Geometry: final body of the model. Coordinates: model frame, mm. Face numbers are marked on the shaded views. A direction names the side the tool comes from. Coordinates: 2 decimals unless noted, no trailing zeros. Write each loop counter-clockwise with the first axis right and the second up, starting at its lowest first coordinate (ties: lowest second). Pieces come first, ordered by that corner, then holes. Notation, with made-up numbers: M -36.5,-38 L -10.5,-38 A25 ccw -10.5,-19 Z; hole C -18.75,31.5 d5. An arc over 180 degrees is marked long. Write item = value, one per line. Start each with the question number.
Item 1: Ray query, L1, parallel to X at y = -152, z = 49.5; L2, parallel to Z at x = 251, y = 7; L3, parallel to Z at x = 23, y = 214. Return the intervals inside material, ascending. Write a range as [from, to].
Item 2: Section A-A on x = -229. Output: boundary loops of the cut face in (y, z), plus the area to 3 significant figures.
Item 3: Reachability of the marked faces 1, 2 and 3 from +Z, -Z, +X, -X, +Y, -Y: full face, straight path, thin tool, end or side. Return the list, or none.
Item 4: First-contact query: pin 1 Ø10 at (y, z) = (1, 39) entering from -X; pin 2 Ø4 at (y, z) = (-86.5, 48) entering from +X; pin 3 Ø8 at (y, z) = (32, 35) entering from -X. Flat tips, straight axial feed; report the tip coordinate or a pass-through.
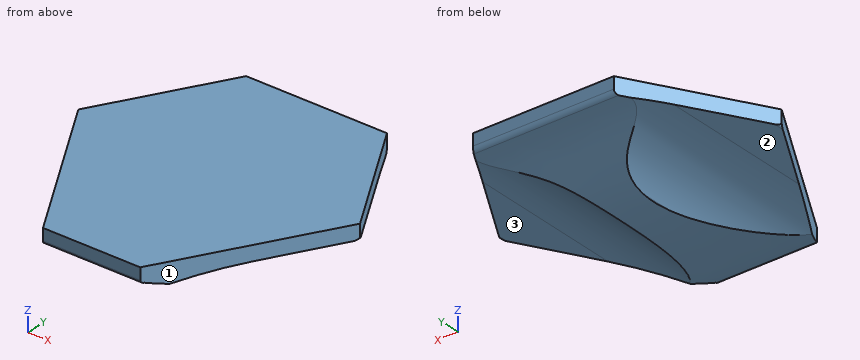
from build123d import *

# Parameters (mm, degrees)
BOSS_EXTRUDE1_DEPTH      = 101.6
BOSS_EXTRUDE1_DEPTH_BACK = 25.4
CUT_EXTRUDE5_DEPTH       = 690.084726286
CUT_EXTRUDE7_START       = -167.47195291
CUT_EXTRUDE7_DEPTH       = 334.94390582


with BuildPart() as part:
    # Sketch2 → Boss-Extrude1 (new, two sides: drawn at the far end of the back side and taken through both)
    with BuildSketch(Plane.XY.offset(-BOSS_EXTRUDE1_DEPTH_BACK)):
        Polygon((-152.4, 263.964543073), (152.4, 263.964543073), (304.8, 0), (105.247275902, -345.635456927), (-105.247275902, -345.635456927), (-304.8, 0), align=None)
    extrude(amount=BOSS_EXTRUDE1_DEPTH + BOSS_EXTRUDE1_DEPTH_BACK)

    # Sketch3 → Cut-Extrude5 (cut, through all)
    with BuildSketch(Plane(origin=(0, 263.964543073, 0), x_dir=(1, 0, 0), z_dir=(0, 1, 0))):
        with BuildLine():
            Line((-304.8, -76.2), (-304.8, 25.4))
            Line((-304.8, 25.4), (304.8, 25.4))
            Line((304.8, 25.4), (304.8, -76.2))
            ThreePointArc((304.8, -76.2), (302.940128061, -71.709871939), (298.45, -69.85))
            ThreePointArc((298.45, -69.85), (252.51979015, -69.714637969), (206.591176001, -69.30855658))
            ThreePointArc((206.591176001, -69.30855658), (119.939950937, -53.691572752), (43.155890442, -10.604068265))
            ThreePointArc((43.155890442, -10.604068265), (34.818219716, -4.738506069), (25.792249783, 0))
            ThreePointArc((25.792249783, 0), (0, 5.478791422), (-25.792249783, 0))
            ThreePointArc((-25.792249783, 0), (-34.818219716, -4.738506069), (-43.155890442, -10.604068265))
            ThreePointArc((-43.155890442, -10.604068265), (-119.939950937, -53.691572752), (-206.591176001, -69.30855658))
            ThreePointArc((-206.591176001, -69.30855658), (-252.51979015, -69.714637969), (-298.45, -69.85))
            ThreePointArc((-298.45, -69.85), (-302.940128061, -71.709871939), (-304.8, -76.2))
        make_face()
    extrude(amount=-CUT_EXTRUDE5_DEPTH, mode=Mode.SUBTRACT)

    # Cut-Extrude7: read off the stored shape, not the designer's step
    # Cut-Extrude7 outline → Cut-Extrude7 (cut)
    with BuildSketch(Plane(origin=(0, 0, 0), x_dir=(0, 0, -1), z_dir=(1, 0, 0)).offset(CUT_EXTRUDE7_START)):
        with BuildLine():
            ThreePointArc((-76.2, 263.964543073), (-69.788494044, 261.94466991), (-65.692525933, 256.614534691))
            add(Edge.make_bspline(
                [(-65.692525933, 256.614534691), (-71.486350731, 90.510366485), (-0.882192536, 198.749340281), (23.113391949, 17.574151868), (-16.69864439, -54.274132463), (-38.1, -256.513950378), (-69.85, -339.285456927)],
                knots=[0, 0, 0, 0, 0, 0, 0, 1, 1, 1, 1, 1, 1, 1], degree=6))
            ThreePointArc((-69.85, -339.285456927), (-71.709871939, -343.775584987), (-76.2, -345.635456927))
            Line((-76.2, -345.635456927), (7, -345.635456927))
            Line((7, -345.635456927), (7, 263.964543073))
            Line((7, 263.964543073), (-76.2, 263.964543073))
        make_face()
    extrude(amount=CUT_EXTRUDE7_DEPTH, mode=Mode.SUBTRACT)


solid = part.part
Responses:
q1.L1 = [-109.03, 109.03]
q1.L2 = [69.71, 101.6]
q1.L3 = [64.69, 101.6]
q2.outline = M -131.29,69.54 L 131.29,69.54 L 131.29,101.6 L -131.29,101.6 Z
q2.area = 8,420 mm²
q3.face_1 = +Z, -Z, +X, -Y
q3.face_2 = -Z, -X, +Y, -Y
q3.face_3 = -Z, +X, +Y, -Y
q4.pin_1 = -96.53
q4.pin_2 = 110.26
q4.pin_3 = -86.48
